Answer from the drawing. Dimensions are ordinates in mm from the lowest x, y and z of the part. Give positions to 0.01 mm unless a question says otherwise; leave off trailing zeros. Write each loop counter-clockwise with the first axis right and the second up, starting at its lowest first coordinate (ties: lowest second). Pieces come first, ordered by that corner, then holes.
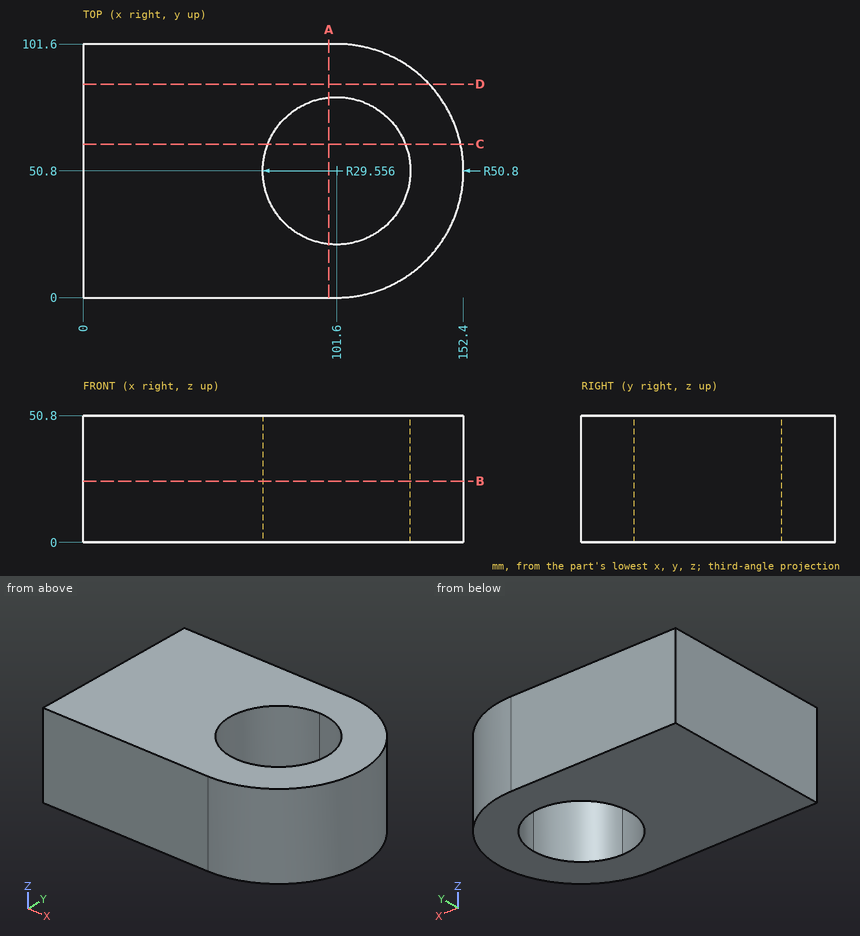
Item 1: Each of these flat-tipped pins is pushed along its axis until it touches: P1, Ø1, axis at y = 49.5, z = 32, coming from the +X side; P2, Ø6, axis at y = 64.5, z = 20.5, coming from the +X side. Where does it stop, or does it pass through?
Conclusion:
P1: stops at x = 152.39
P2: stops at x = 151.26
Item 2: A cutting plane is placed at A-A, the plane x = 98.5. Give the vertices of the cut face in (y, z), plus the area to 4 significant figures.
Conclusion:
outline: (0, 0) - (21.41, 0) - (21.41, 50.8) - (0, 50.8) - close; (80.19, 0) - (101.6, 0) - (101.6, 50.8) - (80.19, 50.8) - close
area: 2,175 mm2
Item 3: Consider probe 1 along X at (y, z) = (46.5, 32); probe 2 along Y at (x, z) = (103.5, 14) (1 decimal); probe 3 along Y at (x, z) = (75, 11.5) (1 decimal). Determine where each line is inside the solid, lowest interval first.
Conclusion:
probe 1: x = 0 to 72.36, 130.84 to 152.22
probe 2: y = 0 to 21.3, 80.3 to 101.6
probe 3: y = 0 to 37.9, 63.7 to 101.6
Item 4: A cutting plane is placed at B-B, the plane z = 24.5. Give the vertices of the cut face in (x, y).
Conclusion:
outline: (0, 0) - (101.6, 0) arc R50.8 ccw to (101.6, 101.6) - (0, 101.6) - close; hole circle Ø59.11 at (101.6, 50.8)
Item 5: A cutting plane is placed at C-C, the plane y = 61.5. Give the vertices of the cut face in (x, z).
Conclusion:
outline: (0, 0) - (74.05, 0) - (74.05, 50.8) - (0, 50.8) - close; (129.15, 0) - (151.26, 0) - (151.26, 50.8) - (129.15, 50.8) - close
Item 6: A cutting plane is placed at D-D, the plane y = 85.5. Give the vertices of the cut face in (x, z), plus the area to 3 significant figures.
Conclusion:
outline: (0, 0) - (138.7, 0) - (138.7, 50.8) - (0, 50.8) - close
area: 7,050 mm2
